from build123d import *

# Parameters (mm, degrees)
F1_DEPTH  = 19.812
F2_R      = 7.9410723376
F3_DEPTH  = 53.594
F4_DEPTH  = 72.136
F5_W      = 80.0100006163
F5_H      = 27.649730444
F6_DEPTH  = 41.148
F8_DEPTH  = 64.516
F10_DEPTH = 9.652
F12_DEPTH = 9.144
F13_R     = 5.2636855274
F14_DEPTH = 114.046


with BuildPart() as f1:
    # F0 (on Top) → F1 (new body)
    with BuildSketch(Plane.XY):
        with BuildLine():
            Line((62.7238675952, 24.0631569177), (60.7514679523, 24.0631569177))
            ThreePointArc((60.7514679523, 24.0631569177), (38.7298974086, 0.1503936946), (60.7514679523, -23.7623695284))
            Line((60.7514679523, -23.7623695284), (62.7238675952, -23.7623695284))
            Line((62.7238675952, -23.7623695284), (62.7238675952, 24.0631569177))
        make_face()
        with BuildLine():
            Line((60.7514679523, 24.0631569177), (-54.584030062, 24.0631569177))
            Line((-54.584030062, 24.0631569177), (-54.584030062, 23.9759786156))
            ThreePointArc((-54.584030062, 23.9759786156), (-37.7367973986, 16.997626358), (-30.758445141, 0.1503936946))
            ThreePointArc((-30.758445141, 0.1503936946), (-37.7367973986, -16.6968389687), (-54.584030062, -23.6751912263))
            Line((-54.584030062, -23.6751912263), (-54.584030062, -23.7623695284))
            Line((-54.584030062, -23.7623695284), (60.7514679523, -23.7623695284))
            ThreePointArc((60.7514679523, -23.7623695284), (38.7298974086, 0.1503936946), (60.7514679523, 24.0631569177))
        make_face()
        with BuildLine():
            Line((-54.584030062, -23.6751912263), (-54.584030062, 23.9759786156))
            ThreePointArc((-54.584030062, 23.9759786156), (-78.4096149829, 0.1503936946), (-54.584030062, -23.6751912263))
        make_face()
        with BuildLine():
            ThreePointArc((86.7178377817, 0.1503936946), (78.9778656739, 17.8002705149), (60.7514679523, 24.0631569177))
            Line((60.7514679523, 24.0631569177), (62.7238675952, 24.0631569177))
            Line((62.7238675952, 24.0631569177), (62.7238675952, -23.7623695284))
            Line((62.7238675952, -23.7623695284), (60.7514679523, -23.7623695284))
            ThreePointArc((60.7514679523, -23.7623695284), (78.9778656739, -17.4994831256), (86.7178377817, 0.1503936946))
        make_face()
        with BuildLine():
            ThreePointArc((-30.758445141, 0.1503936946), (-37.7367973986, 16.997626358), (-54.584030062, 23.9759786156))
            Line((-54.584030062, 23.9759786156), (-54.584030062, -23.6751912263))
            ThreePointArc((-54.584030062, -23.6751912263), (-37.7367973986, -16.6968389687), (-30.758445141, 0.1503936946))
        make_face()
    extrude(amount=-F1_DEPTH)

    # F2 (on face) → F3 (cut)
    with BuildSketch(Plane.XY):
        with Locations((-64.4258856773, 0)):
            Circle(F2_R)
    extrude(amount=-F3_DEPTH, mode=Mode.SUBTRACT)

    # F2 (on face) → F4 (cut)
    with BuildSketch(Plane.XY):
        with Locations((-64.4258856773, 0)):
            Circle(F2_R)
        with Locations((64.4258856773, 0)):
            Circle(F2_R)
    extrude(amount=-F4_DEPTH, mode=Mode.SUBTRACT)

    # F5 (on face) → F6 (join)
    with BuildSketch(Plane.XY):
        with Locations((4.7556925565, 1.4888346195)):
            Rectangle(F5_W, F5_H)
    extrude(amount=F6_DEPTH)

    # F7 (on face) → F8 (cut)
    with BuildSketch(Plane.XZ.offset(12.3360306025)):
        with BuildLine():
            Line((-25.8717667552, 41.148), (35.3831518682, 41.148))
            ThreePointArc((35.3831518682, 41.148), (4.7556925565, 71.7754593117), (-25.8717667552, 41.148))
        make_face()
        with BuildLine():
            ThreePointArc((-25.8717667552, 41.148), (4.7556925565, 10.5205406883), (35.3831518682, 41.148))
            Line((35.3831518682, 41.148), (-25.8717667552, 41.148))
        make_face()
    extrude(amount=-F8_DEPTH, mode=Mode.SUBTRACT)

    # F9 (on face) → F10 (join)
    with BuildSketch(Plane(origin=(-35.2493077517, 0, 0), x_dir=(0, -1, 0), z_dir=(-1, 0, 0))):
        with BuildLine():
            Line((-14.9469008146, 41.148), (11.9692315755, 41.148))
            ThreePointArc((11.9692315755, 41.148), (-1.4888346195, 54.606066195), (-14.9469008146, 41.148))
        make_face()
    extrude(amount=-F10_DEPTH)

    # F11 (on face) → F12 (join)
    with BuildSketch(Plane.YZ.offset(44.7606928647)):
        with BuildLine():
            Line((-12.0193907988, 41.148), (14.9970600378, 41.148))
            ThreePointArc((14.9970600378, 41.148), (1.4888346195, 54.6562254183), (-12.0193907988, 41.148))
        make_face()
    extrude(amount=-F12_DEPTH)

    # F13 (on face) → F14 (cut)
    with BuildSketch(Plane.YZ.offset(44.7606928647)):
        with Locations((1.4888346195, 41.148)):
            Circle(F13_R)
    extrude(amount=-F14_DEPTH, mode=Mode.SUBTRACT)


solid = f1.part
Could you check a few things on this model? Use its own coordinates, in mm. A direction names the side the tool comes from. Coordinates: 2 decimals unless noted, no trailing zeros. Order: outer loops, then holes, each group sorted by start corner. A loop starts at its lowest first (then second) coordinate and runs counter-clockwise, first axis right, second up. Notation, with made-up numbers: (82.5, -27.5) - (136.5, -27.5) arc R24 cw to (136.5, 4.5) - close; hole circle Ø7 at (34, -27.75). An arc over 180 degrees is marked (long way). Answer in a Markdown table with one row per item. Add a question column.
(1) Will these pins go through, and if not, where does the flat tip stop? pin 1 (1 mm diameter, centred on x = 36, z = -2.5, fed in from -Y); pin 2 (12.5 mm diameter, centred on x = -4, z = 12.5, fed in from +Y); pin 3 (7 mm diameter, centred on x = 40, y = 11, fed in from +Z) (3 decimals).
(2) On a 3-axis mill with a long thin cutter (end or side, diameter ignored), from which of +Z, -Z, +X, -X, +Y, -Y can I reach the whole of each face in a straight line? I mean faces 1 (the face through (-35.249, 2, 28)), 2 (the face through (-25.597, 2, 48)), 3 (the face through (44.761, 1, 27)). Say none if no direction works.
(3) If we section it at B-B, the plane x = 58: Please give me the cut outline in (y, z), then the cut area to 3 significant figures.
(4) If we mould it in two halves opening along Y, with no side actions, what happens to faces 4 (the face through (-56.852, 2.385, -9.767)), 5 (the face through (4, -12.336, 7)), 6 (the face through (-30.491, 1.193, 54.603))? For each: released by +Y, released by -Y, zero draft, split by the parting line, or undercut.
(5) If we section it at A-A, the plane z = -8: Please give me the cut outline in (x, y), then the cut area to 3 significant figures.
(6) I need wall thicknesses on L1, parallel to Y at x = -23.5, z = 7; L2, parallel to Z at x = 53.5, y = 10; L3, parallel to Y at x = 23.5, z = -14. Which ranges of each line are inside material? Lowest first, please.
(7) If we section it at D-D, the plane z = 13.5: Please give me the cut outline in (x, y), then the cut area to 3 significant figures.
Results are:
| question | item | result |
|---|---|---|
| 1 | pin 1 | stops at y = -23.76 |
| 1 | pin 2 | stops at y = 15.31 |
| 1 | pin 3 | stops at z = 53.245 |
| 2 | face 1 | +Z, -X, +Y, -Y |
| 2 | face 2 | +Z, +Y, -Y |
| 2 | face 3 | +Z, +X, +Y, -Y |
| 3 | outline | (-23.76, -19.81) - (-4.67, -19.81) - (-4.67, 0) - (-23.76, 0) - close; (4.67, -19.81) - (24.06, -19.81) - (24.06, 0) - (4.67, 0) - close |
| 3 | area | 763 mm2 |
| 4 | face 4 | undercut |
| 4 | face 5 | released by -Y |
| 4 | face 6 | split by the parting line |
| 5 | outline | (-54.58, -23.76) - (60.75, -23.76) arc R23.99 ccw (long way) to (60.75, 24.06) - (-54.58, 24.06) - (-54.58, 23.98) arc R23.83 ccw to (-54.58, -23.68) - close; hole circle Ø15.88 at (-64.43, 0); hole circle Ø15.88 at (64.43, 0) |
| 5 | area | 7,010 mm2 |
| 6 | L1 | y = -12.34 to 15.31 |
| 6 | L2 | z = -19.81 to 0 |
| 6 | L3 | y = -23.76 to 24.06 |
| 7 | outline | (-35.25, -12.34) - (-8.42, -12.34) - (-8.42, 15.31) - (-35.25, 15.31) - close; (17.93, -12.34) - (44.76, -12.34) - (44.76, 15.31) - (17.93, 15.31) - close |
| 7 | area | 1,480 mm2 |
